Could you check a few things on this model? Use its own coordinates, in mm. Give positions to 0.01 mm unless a question says otherwise; leave off trailing zeros. Write each loop counter-clockwise with the first axis right and the second up, starting at its lowest first coordinate (ties: lowest second). Pieces come first, ordered by that corner, then holes. Notation, with made-up numbers: (10.5, 63.5) -> (41.5, 63.5) arc R26 cw to (41.5, 101.5) -> close; hole circle Ø4 at (-38, 82). An arc over 180 degrees is marked (long way). Write item = value, one per line. Start each with the question number.
```python
from build123d import *

# Parameters (mm, degrees)
SKETCH1_R           = 12.5
BOSS_EXTRUDE1_DEPTH = 6
M3_TAPPED_HOLE1_D   = 2.5


with BuildPart() as part:
    # Sketch1 → Boss-Extrude1 (new body)
    with BuildSketch(Plane(origin=(0, 0, 0), x_dir=(1, 0, 0), z_dir=(0, 1, 0))):
        with Locations(Location((0, 0, 0), (0, 0, 270))):
            Circle(SKETCH1_R)
        with BuildLine():
            Line((-0.25, 4.993746089), (-0.476626074, 3.971501931))
            ThreePointArc((-0.476626074, 3.971501931), (-0.890083736, 3.899711649), (-1.293744854, 3.784999901))
            Line((-1.293744854, 3.784999901), (-1.941463008, 4.607680695))
            ThreePointArc((-1.941463008, 4.607680695), (-2.169418696, 4.50484434), (-2.391947442, 4.390738825))
            Line((-2.391947442, 4.390738825), (-2.152595362, 3.371399295))
            ThreePointArc((-2.152595362, 3.371399295), (-2.493959207, 3.12732593), (-2.807873746, 2.848832222))
            Line((-2.807873746, 2.848832222), (-3.748395457, 3.30900763))
            ThreePointArc((-3.748395457, 3.30900763), (-3.909157412, 3.117449009), (-4.060140358, 2.918091889))
            Line((-4.060140358, 2.918091889), (-3.402216738, 2.103549682))
            ThreePointArc((-3.402216738, 2.103549682), (-3.603875472, 1.735534956), (-3.765868806, 1.348418382))
            Line((-3.765868806, 1.348418382), (-4.812912215, 1.354945022))
            ThreePointArc((-4.812912215, 1.354945022), (-4.874639561, 1.11260467), (-4.924172682, 0.867481066))
            Line((-4.924172682, 0.867481066), (-3.977987365, 0.419066256))
            ThreePointArc((-3.977987365, 0.419066256), (-4, 0), (-3.977987365, -0.419066256))
            Line((-3.977987365, -0.419066256), (-4.924172682, -0.867481066))
            ThreePointArc((-4.924172682, -0.867481066), (-4.874639561, -1.11260467), (-4.812912215, -1.354945022))
            Line((-4.812912215, -1.354945022), (-3.765868806, -1.348418382))
            ThreePointArc((-3.765868806, -1.348418382), (-3.603875472, -1.735534956), (-3.402216738, -2.103549682))
            Line((-3.402216738, -2.103549682), (-4.060140358, -2.918091889))
            ThreePointArc((-4.060140358, -2.918091889), (-3.909157412, -3.117449009), (-3.748395457, -3.30900763))
            Line((-3.748395457, -3.30900763), (-2.807873746, -2.848832222))
            ThreePointArc((-2.807873746, -2.848832222), (-2.493959207, -3.12732593), (-2.152595362, -3.371399295))
            Line((-2.152595362, -3.371399295), (-2.391947442, -4.390738825))
            ThreePointArc((-2.391947442, -4.390738825), (-2.169418696, -4.50484434), (-1.941463008, -4.607680695))
            Line((-1.941463008, -4.607680695), (-1.293744854, -3.784999901))
            ThreePointArc((-1.293744854, -3.784999901), (-0.890083736, -3.899711649), (-0.476626074, -3.971501931))
            Line((-0.476626074, -3.971501931), (-0.25, -4.993746089))
            ThreePointArc((-0.25, -4.993746089), (0, -5), (0.25, -4.993746089))
            Line((0.25, -4.993746089), (0.476626074, -3.971501931))
            ThreePointArc((0.476626074, -3.971501931), (0.890083736, -3.899711649), (1.293744854, -3.784999901))
            Line((1.293744854, -3.784999901), (1.941463008, -4.607680695))
            ThreePointArc((1.941463008, -4.607680695), (2.169418696, -4.50484434), (2.391947442, -4.390738825))
            Line((2.391947442, -4.390738825), (2.152595362, -3.371399295))
            ThreePointArc((2.152595362, -3.371399295), (2.493959207, -3.12732593), (2.807873746, -2.848832222))
            Line((2.807873746, -2.848832222), (3.748395457, -3.30900763))
            ThreePointArc((3.748395457, -3.30900763), (3.909157412, -3.117449009), (4.060140358, -2.918091889))
            Line((4.060140358, -2.918091889), (3.402216738, -2.103549682))
            ThreePointArc((3.402216738, -2.103549682), (3.603875472, -1.735534956), (3.765868806, -1.348418382))
            Line((3.765868806, -1.348418382), (4.812912215, -1.354945022))
            ThreePointArc((4.812912215, -1.354945022), (4.874639561, -1.11260467), (4.924172682, -0.867481066))
            Line((4.924172682, -0.867481066), (3.977987365, -0.419066256))
            ThreePointArc((3.977987365, -0.419066256), (4, 0), (3.977987365, 0.419066256))
            Line((3.977987365, 0.419066256), (4.924172682, 0.867481066))
            ThreePointArc((4.924172682, 0.867481066), (4.874639561, 1.11260467), (4.812912215, 1.354945022))
            Line((4.812912215, 1.354945022), (3.765868806, 1.348418382))
            ThreePointArc((3.765868806, 1.348418382), (3.603875472, 1.735534956), (3.402216738, 2.103549682))
            Line((3.402216738, 2.103549682), (4.060140358, 2.918091889))
            ThreePointArc((4.060140358, 2.918091889), (3.909157412, 3.117449009), (3.748395457, 3.30900763))
            Line((3.748395457, 3.30900763), (2.807873746, 2.848832222))
            ThreePointArc((2.807873746, 2.848832222), (2.493959207, 3.12732593), (2.152595362, 3.371399295))
            Line((2.152595362, 3.371399295), (2.391947442, 4.390738825))
            ThreePointArc((2.391947442, 4.390738825), (2.169418696, 4.50484434), (1.941463008, 4.607680695))
            Line((1.941463008, 4.607680695), (1.293744854, 3.784999901))
            ThreePointArc((1.293744854, 3.784999901), (0.890083736, 3.899711649), (0.476626074, 3.971501931))
            Line((0.476626074, 3.971501931), (0.25, 4.993746089))
            ThreePointArc((0.25, 4.993746089), (0, 5), (-0.25, 4.993746089))
        make_face(mode=Mode.SUBTRACT)
    extrude(amount=BOSS_EXTRUDE1_DEPTH)

    # M3 Tapped Hole1 (through all)
    with Locations(Plane(origin=(0, 6, 0), x_dir=(1, 0, 0), z_dir=(0, 1, 0))):
        with Locations((0, 9), (7.794228634, 4.5), (7.794228634, -4.5), (0, -9), (-7.794228634, -4.5), (-7.794228634, 4.5)):
            Hole(M3_TAPPED_HOLE1_D / 2)


solid = part.part
```
(1) I'm going to push flat-ended pins straight in: pin 1 (2 mm diameter, centred on y = 1.5, z = -1.5, fed in from +X); pin 2 (3 mm diameter, centred on y = 2, z = 6, fed in from -X); pin 3 (1 mm diameter, centred on x = -6.5, y = 2.5, fed in from -Z). Where does each tip first touch, or does it pass through?
(2) Imagine slicing it at C-C (y = 4.65). State how many separate pieces and enclosed holes the cut face has, then the cut area to 3 significant figures.
(3) Imagine slicing it at B-B (x = -8.5). Please give me the cut outline in (y, z), then the cut area to 3 significant figures.
(4) Imagine slicing it at A-A (z = 0). Please give me the cut outline in (x, y), then the cut area to 3 significant figures.
(5) If I drill on line 1 along X through (y, z) = (4.3, -4.5); line 2 along X through (y, z) = (5.1, 0.5); line 3 along X through (y, z) = (3.55, -9), over which ranges is the centre line in solid material (lowest first)? Write a range as from..to.
(6) Imagine slicing it at D-D (z = -9). Please give me the cut outline in (x, y), then the cut area to 3 significant figures.
(7) We'd pull the mould along X, two halves only. Please class faces 1 (the cylindrical face through (3.755, 2.958, 11.923)), 2 (the flat face through (3.272, 2.958, 3.076)), 3 (the flat face through (-5, 6, 0)): released by +X, released by -X, zero draft, split by the parting line, or undercut.
Answers below:
q1.pin_1 = 12.49
q1.pin_2 = -11.66
q1.pin_3 = -10.97
q2.separate_pieces = 1
q2.enclosed_holes = 7
q2.area = 401 mm^2
q3.outline = (0, -9.17) -> (6, -9.17) -> (6, -5.53) -> (0, -5.53) -> close; (0, -3.47) -> (6, -3.47) -> (6, 3.47) -> (0, 3.47) -> close; (0, 5.53) -> (6, 5.53) -> (6, 9.17) -> (0, 9.17) -> close
q3.area = 85.2 mm^2
q4.outline = (-12.5, 0) -> (-4, 0) -> (-4, 6) -> (-12.5, 6) -> close; (4, 0) -> (12.5, 0) -> (12.5, 6) -> (4, 6) -> close
q4.area = 102 mm^2
q5.line_1 = -11.66..-9.04, -6.54..-2.18, -1.86..-0.36, 0.36..1.86, 2.18..6.54, 9.04..11.66
q5.line_2 = -12.49..-4.15, 4.15..12.49
q5.line_3 = -8.67..-1.25, 1.25..8.67
q6.outline = (-8.67, 0) -> (-1.25, 0) -> (-1.25, 6) -> (-8.67, 6) -> close; (1.25, 0) -> (8.67, 0) -> (8.67, 6) -> (1.25, 6) -> close
q6.area = 89.1 mm^2
q7.face_1 = split by the parting line
q7.face_2 = undercut
q7.face_3 = zero draft
